CAD build for the part. Positions are in the model's coordinates, mm. Face numbers are marked on the shaded views. A direction names the side the tool comes from. Coordinates: 2 decimals unless noted, no trailing zeros. Order: outer loops, then holes, each group sorted by start corner. A loop starts at its lowest first (then second) coordinate and runs counter-clockwise, first axis right, second up. Notation, with made-up numbers: M 3,84 L 57,84 A26 ccw 57,105 Z; hole C 17,83 d2. An arc over 180 degrees is marked long. One line per item, written item: value.
from build123d import *

# Parameters (mm, degrees)
SKETCH2_R          = 1.25
CUT_EXTRUDE1_DEPTH = 22.512750464


with BuildPart() as part:
    # Sketch1 → Revolve1 (revolve)
    with BuildSketch(Plane(origin=(0, 0, 0), x_dir=(1, 0, 0), z_dir=(0, 1, 0))):
        Polygon((-12.563694364, 14.55), (-12.563694364, 16.55), (4.186305636, 16.55), (4.186305636, 18.55), (5.686305636, 18.55), (5.686305636, 15.537968137), (4.955330367, 15.537968137), (8.9490561, 12.528479936), (8.9490561, 6), (6.936305636, 6), (6.936305636, 11.540924884), (2.943128086, 14.55), align=None)
    revolve(axis=Axis((-37.278866169, 0, 0), (1, 0, 0)))

    # Sketch2 → Cut-Extrude1 (cut, through all)
    with BuildSketch(Plane(origin=(8.9490561, 0, 0), x_dir=(0, 0, -1), z_dir=(1, 0, 0))):
        with Locations((0, 9)):
            Circle(SKETCH2_R)
        with Locations((6.363961031, 6.363961031)):
            Circle(SKETCH2_R)
        with Locations((9, 0)):
            Circle(SKETCH2_R)
        with Locations((6.363961031, -6.363961031)):
            Circle(SKETCH2_R)
        with Locations((0, -9)):
            Circle(SKETCH2_R)
        with Locations((-6.363961031, -6.363961031)):
            Circle(SKETCH2_R)
        with Locations((-9, 0)):
            Circle(SKETCH2_R)
        with Locations((-6.363961031, 6.363961031)):
            Circle(SKETCH2_R)
    extrude(amount=-CUT_EXTRUDE1_DEPTH, mode=Mode.SUBTRACT)


solid = part.part
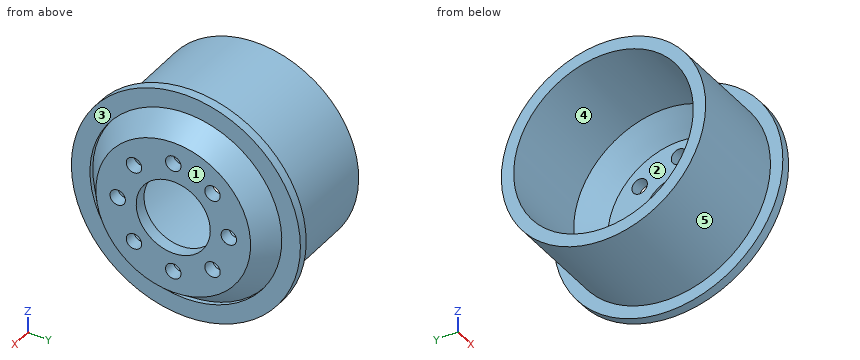
Q1. Slice it at A-A (z = 0). Give the number of separate pieces and of enclosed holes in the cut face, plus the area to 3 significant figures.
Recorded:
separate pieces: 4
enclosed holes: 0
area: 110 mm^2
Q2. Mould opens along Z. For the marked faces 3, 4 and 5 say: released by +Z, released by -Z, zero draft, split by the parting line, or undercut.
Recorded:
face 3: zero draft
face 4: undercut
face 5: split by the parting line
Q3. Drill centre lines: line 1 along Y through (x, z) = (0.25, 0); line 2 along Y through (x, z) = (8.4, 0); line 3 along Z through (x, y) = (-6.75, 0.5). Where is each one in solid material? Low to high.
Recorded:
line 1: y = -16.55 to -14.55, 14.55 to 16.55
line 2: y = -12.94 to -10.25, -7.75 to -6, 6 to 7.75, 10.25 to 12.94
line 3: z = -16.54 to -14.54, 14.54 to 16.54
Q4. Slice it at C-C (x = -7.5). List the corners of the cut face in (y, z).
Recorded:
outline: C 0,0 d33.1; hole C 0,0 d29.1
Q5. Which spindle directions (+Z, -Z, +X, -X, +Y, -Y) get a long thin tool onto all of the face, cutting with end or side? Do the marked faces 1 and 2. Say none if no direction does.
Recorded:
face 1: +Z, -Z, +X, +Y, -Y
face 2: -X
Q6. Pin check, flat tips, straight feed: pin 1 Ø3 at (x, y) = (-6, -10.5) entering from -Z; pin 2 Ø8 at (x, z) = (-4.5, 6.5) entering from +Y; pin 3 Ø3 at (y, z) = (6.36, -6.36) entering from -X. Stop position of each tip, or through.
Recorded:
pin 1: stops at z = -13.89
pin 2: stops at y = 16.36
pin 3: stops at x = 6.94
